Design review of the part built by this model. Coordinates are the model's own, in mm. A direction names the side the tool comes from. Round coordinates to 2 decimals unless told otherwise and drop trailing zeros. Order: outer loops, then holes, each group sorted by start corner. A loop starts at its lowest first (then second) coordinate and runs counter-clockwise, first axis right, second up. Notation, with made-up numbers: (75, 5) - (98, 5) arc R26 ccw to (98, 32) - close; hole circle Ø4 at (-39, 2.25). An arc over 180 degrees is marked (long way). Write item = value, one per line.
Solid Edge part; units mm, degrees
sketch "Sketch1" plane through (0, 0, 0) normal (0, -1, 0) x (1, 0, 0)
  line L0 (8.6, 18.5) -> (8.6, 7.5)
  line L1 (8.6, 7.5) -> (4, 7.5)
  line L2 (4, 7.5) -> (4, 18.5)
  line L3 (4, 18.5) -> (0, 18.5)
  line L4 (0, 18.5) -> (0, 0)
  line L5 (0, 0) -> (12.6, 0)
  line L6 (12.6, 0) -> (12.6, 18.5)
  line L7 (12.6, 18.5) -> (8.6, 18.5)
extrude "Protrusion1" add sketch "Sketch1" along normal blind 10
sketch "Sketch2" plane through (12.6, -5, 7.5) normal (1, 0, 0) x (0, 1, 0)
  circle A0 centre (0, 2.5) radius 1.9
extrude "Cutout1" cut sketch "Sketch2" against normal through all
sketch "Sketch3" plane through (6.3, -5, 0) normal (0, 0, -1) x (1, 0, 0)
  line L0 (-6.3, -5) -> (-11.8616, -2.2393)
  line L1 (-6.3, 5) -> (-11.8616, 2.2393)
  line L2 (-6.3, 5) -> (6.3, 5)
  line L3 (6.3, 5) -> (11.8616, 2.2393)
  line L4 (6.3, -5) -> (11.8616, -2.2393)
  line L5 (-6.3, -5) -> (6.3, -5)
  arc A0 (-11.8616, -2.2393) -> (-11.8616, 2.2393) centre (-10.75, 0) cw
  arc A1 (11.8616, 2.2393) -> (11.8616, -2.2393) centre (10.75, 0) cw
  circle A2 centre (-10.75, 0) radius 0.875
  circle A3 centre (10.75, 0) radius 0.875
extrude "ExtrudedProtrusion_4" add sketch "Sketch3" along normal blind 2.5
sketch "Sketch4" plane through (6.3, -10, 8) normal (0, -1, 0) x (0, 0, -1)
  circle A0 centre (4.25, 0) radius 1.6
extrude "ExtrudedCutout_2" cut sketch "Sketch4" against normal blind 5
1) To check wall thickness, follow L1, parallel to X at y = -5, z = -1.5 (3 decimals); L2, parallel to X at y = -8.5, z = 13.5; L3, parallel to Z at x = 10.5, y = -5. State the ranges of each line that lie inside material, in increasing order. Write a range as from..to.
Findings:
L1 = -6.95..-5.325, -3.575..16.175, 17.925..19.55
L2 = 0..4, 8.6..12.6
L3 = -2.5..8.1, 11.9..18.5
2) Clearance check with flat-ended pins moving along their axes: pin 1 Ø6 at (y, z) = (-4, 10) entering from +X; pin 2 Ø3 at (y, z) = (-7, 15) entering from -X; pin 3 Ø3.5 at (x, y) = (15, -4.5) entering from +Z; pin 4 Ø2.5 at (y, z) = (-5, 10) entering from +X. State where each tip first meets the part, or that it passes through.
Findings:
pin_1 = 12.6
pin_2 = 0
pin_3 = 0
pin_4 = through
3) The part is to be moulded in two halves that separate along Y. For faces 5 (the cylindrical face through (19.55, -5.04, -1.23)), 6 (the flat face through (-2.74, -1.36, -1.23)), 7 (the flat face through (15, -5, 0)), 8 (the cylindrical face through (17.885, -4.737, -1.232)), say which applies: released by +Y, released by -Y, zero draft, split by the parting line, or undercut.
Findings:
face_5 = split by the parting line
face_6 = released by +Y
face_7 = zero draft
face_8 = undercut
4) We need section B-B on z = -0.5. Write out the cut boundary in (x, y) (3 decimals).
Findings:
outline = (-5.562, -7.239) - (0, -10) - (12.6, -10) - (18.162, -7.239) arc R2.5 ccw to (18.162, -2.761) - (12.6, 0) - (0, 0) - (-5.562, -2.761) arc R2.5 ccw to start; hole circle Ø1.75 at (-4.45, -5); hole circle Ø1.75 at (17.05, -5)
5) We need section C-C on y = -4.5. Write out the cut boundary in (x, z), and give its area (3 significant figures).
Findings:
outline = (-6.9, -2.5) - (-5.17, -2.5) - (-5.17, 0) - (-6.9, 0) - close; (-3.73, -2.5) - (16.33, -2.5) - (16.33, 0) - (12.6, 0) - (12.6, 8.17) - (8.6, 8.17) - (8.6, 7.5) - (4, 7.5) - (4, 8.17) - (0, 8.17) - (0, 0) - (-3.73, 0) - close; (0, 11.83) - (4, 11.83) - (4, 18.5) - (0, 18.5) - close; (8.6, 11.83) - (12.6, 11.83) - (12.6, 18.5) - (8.6, 18.5) - close; (17.77, -2.5) - (19.5, -2.5) - (19.5, 0) - (17.77, 0) - close
area = 212 mm^2
6) For faces 1 (the flat face through (6, -5, 7.5)), 2 (the flat face through (12.6, -5, 7)), 3 (the flat face through (0, -5, 7)), 4 (the flat face through (6, -5, 4)), list the 3-axis set-ups (+Z, -Z, +X, -X, +Y, -Y) from which the entire face can be reached by the end or side of a thin tool; tool diameter is ignored.
Findings:
face_1 = +Z, +Y, -Y
face_2 = +Z, +X, +Y, -Y
face_3 = +Z, -X, +Y, -Y
face_4 = -Y
7) We need section D-D on x = 17.05. Write out the cut boundary in (y, z) (3 decimals).
Findings:
outline = (-7.791, -2.5) - (-5.875, -2.5) - (-5.875, 0) - (-7.791, 0) - close; (-4.125, -2.5) - (-2.209, -2.5) - (-2.209, 0) - (-4.125, 0) - close
8) We need section A-A on x = 3.5. Write out the cut boundary in (y, z).
Findings:
outline = (-10, -2.5) - (0, -2.5) - (0, 18.5) - (-10, 18.5) - close; hole circle Ø3.8 at (-5, 10)
